Verification items for the finished model (mm, model axes). Give positions to 0.01 mm unless a question says otherwise; leave off trailing zeros. Write each loop counter-clockwise with the first axis right and the second up, starting at its lowest first coordinate (ties: lowest second). Pieces come first, ordered by that corner, then holes. Notation, with made-up numbers: M 53,-13.75 L 70,-13.75 A23 cw 70,7.25 Z; hole C 88,3.25 d1. An arc over 180 degrees is marked long. Answer as a JSON object with one key per item and string values.
```python
from build123d import *

# Parameters (mm, degrees)
ESQUISSE1_W        = 250
ESQUISSE1_H        = 250
BOSS_EXTRU_1_DEPTH = 1.5


with BuildPart() as part:
    # Esquisse1 → Boss.-Extru.1 (new body)
    with BuildSketch(Plane.XY):
        with Locations((125, 125)):
            Rectangle(ESQUISSE1_W, ESQUISSE1_H)
        Polygon((24, 20), (170, 20), (170, 150), (24, 150), (24, 155.5), (20, 155.5), (20, 150), (20, 20), (20, 14.5), (24, 14.5), align=None, mode=Mode.SUBTRACT)
    extrude(amount=BOSS_EXTRU_1_DEPTH)


solid = part.part
```
1) Section check A-A on z = 0.95. Record the boundary of the cut face in (x, y), and give its area (3 significant figures).
Completed:
{"outline": "M 0,0 L 250,0 L 250,250 L 0,250 Z; hole M 20,14.5 L 24,14.5 L 24,20 L 170,20 L 170,150 L 24,150 L 24,155.5 L 20,155.5 Z", "area": "43,000 mm2"}
2) Section check C-C on x = 136.5. Record the boundary of the cut face in (y, z).
Completed:
{"outline": "M 0,0 L 20,0 L 20,1.5 L 0,1.5 Z; M 150,0 L 250,0 L 250,1.5 L 150,1.5 Z"}
3) Go/stop test with a flat-tipped pin: pin 1 (10 mm diameter, centred on x = 29.5, y = 124.5, fed in from -Z). Record where the tip stops, or that it passes through.
Completed:
{"pin 1": "passes through"}
4) Section check B-B on y = 118.5. Record the boundary of the cut face in (x, z), and give its area (3 significant figures).
Completed:
{"outline": "M 0,0 L 20,0 L 20,1.5 L 0,1.5 Z; M 170,0 L 250,0 L 250,1.5 L 170,1.5 Z", "area": "150 mm2"}
5) Thickness scan on L1, parallel to Y at x = 48, z = 1.05; L2, parallel to Y at x = 23.5, z = 1.1; L3, parallel to X at y = 60, z = 0.35. Record the ranges inside material, lowest first.
Completed:
{"L1": "y = 0 to 20, 150 to 250", "L2": "y = 0 to 14.5, 155.5 to 250", "L3": "x = 0 to 20, 170 to 250"}
